from build123d import *

# Parameters (mm, degrees)
SKETCH_1_W                 = 7.2
SKETCH_1_H                 = 20
EXTRUDE_1_DEPTH            = 200
SKETCH_2_W                 = 5.7
SKETCH_2_H                 = 14.7
CUT_EXTRUDE_1_DEPTH        = 200
PATTERN_LINEAR_1_COUNT     = 2
PATTERN_LINEAR_1_PITCH     = 185
PATTERN_LINEAR_1_COL_COUNT = 2
PATTERN_LINEAR_1_COL_PITCH = 185


with BuildPart() as part:
    # 草图1 → 凸台-拉伸1 (new, symmetric)
    with BuildSketch(Plane.XY):
        Rectangle(SKETCH_1_W, SKETCH_1_H)
    extrude(amount=EXTRUDE_1_DEPTH, both=True)

    # 草图2 → 切除-拉伸1 (cut, symmetric)
    with BuildSketch(Plane.XY):
        with Locations((0.75, 0)):
            Rectangle(SKETCH_2_W, SKETCH_2_H)
    extrude(amount=CUT_EXTRUDE_1_DEPTH, both=True, mode=Mode.SUBTRACT)

    # 草图4 → 切除-旋转1 (revolve, cut)
    with BuildSketch(Plane.XY, mode=Mode.PRIVATE) as cut_revolve_1_sk:
        Polygon((-3.6, 1.75), (-3.35, 1.75), (-2.1, 3), (-2.1, 0), (-3.6, 0), align=None)
    cut_revolve_1 = revolve(cut_revolve_1_sk.sketch.rotate(Axis((-2.1, 0, 0), (-1, 0, 0)), 90), axis=Axis((-2.1, 0, 0), (-1, 0, 0)), mode=Mode.SUBTRACT)

    # 阵列(线性)1: 切除-旋转1 ×2
    with Locations(*[(0, 0, -i * PATTERN_LINEAR_1_PITCH) for i in range(1, PATTERN_LINEAR_1_COUNT)]):
        add(cut_revolve_1, mode=Mode.SUBTRACT)

    # 阵列(线性)1 col: 切除-旋转1 ×2
    with Locations(*[(0, 0, i * PATTERN_LINEAR_1_COL_PITCH) for i in range(1, PATTERN_LINEAR_1_COL_COUNT)]):
        add(cut_revolve_1, mode=Mode.SUBTRACT)


solid = part.part
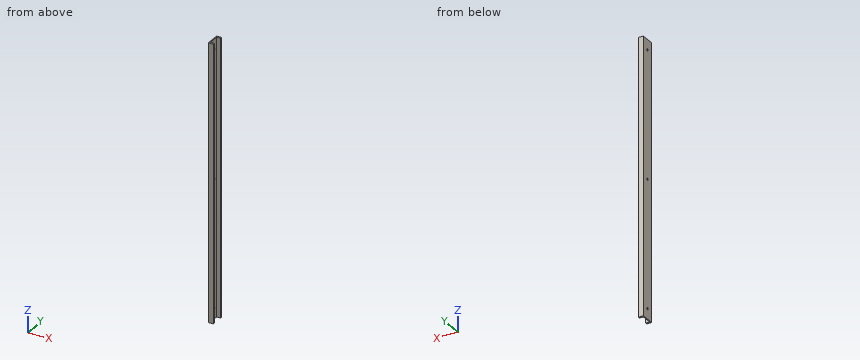
Input: part model. Units: mm. Frame: model coordinates. Coordinates: 2 decimals unless noted, no trailing zeros. Order: outer loops, then holes, each group sorted by start corner. A loop starts at its lowest first (then second) coordinate and runs counter-clockwise, first axis right, second up. Notation, with made-up numbers: M -9,0.25 L 38,0.25 A33 ccw 38,31.25 Z; hole C 8,-22 d10. An arc over 180 degrees is marked long. Answer in a Markdown table with one row per item.
(1) Contact query for flat-ended pins moving along their axis: pin 1 Ø1 at (y, z) = (2, 16.5) entering from +X; pin 2 Ø3 at (y, z) = (0, 185) entering from -X; pin 3 Ø5.5 at (y, z) = (0, -185) entering from +X; pin 4 Ø4 at (y, z) = (0, 0) entering from +X. Output: stop coordinate, or through.
Numbers:
| item | result |
|---|---|
| pin 1 | stops at x = -2.1 |
| pin 2 | passes through |
| pin 3 | stops at x = -2.35 |
| pin 4 | stops at x = -3.1 |
(2) Section query B-B, the plane z = -58. Output: boundary loops of the cut face in (x, y).
Numbers:
| item | result |
|---|---|
| outline | M -3.6,-10 L 3.6,-10 L 3.6,-7.35 L -2.1,-7.35 L -2.1,7.35 L 3.6,7.35 L 3.6,10 L -3.6,10 Z |
(3) Material intervals for line 1 (Y direction, x = 1.25, z = 16.5); line 2 (X direction, y = -4.5, z = 101.5), sorted ascending. Write a range as [from, to].
Numbers:
| item | result |
|---|---|
| line 1 | y = [-10, -7.35], [7.35, 10] |
| line 2 | x = [-3.6, -2.1] |
(4) Section query A-A, the plane x = 1.5. Output: boundary loops of the cut face in (y, z).
Numbers:
| item | result |
|---|---|
| outline | M -10,-200 L -7.35,-200 L -7.35,200 L -10,200 Z; M 7.35,-200 L 10,-200 L 10,200 L 7.35,200 Z |
